```python
from build123d import *

# Parameters (mm, degrees)
SKETCH_1_R          = 0.9
SKETCH_1_W          = 6
SKETCH_1_H          = 8
EXTRUDE_1_DEPTH     = 16.3
SKETCH_2_R          = 0.75
CUT_EXTRUDE_1_DEPTH = 4
CUT_EXTRUDE_START   = -16
SKETCH_2_3_R        = 0.75
CUT_EXTRUDE_2_DEPTH = 4


with BuildPart() as part:
    # 草图1 → 凸台-拉伸1 (new body)
    # profile 1 of 4: a face of its own
    with BuildSketch(Plane.XY):
        Polygon((44, 10), (0, 10), (0, 4), (5, 4), (11, 4), (33, 4), (39, 4), (44, 4), align=None)
        with Locations((8, 7)):
            Circle(SKETCH_1_R, mode=Mode.SUBTRACT)
        with Locations((36, 7)):
            Circle(SKETCH_1_R, mode=Mode.SUBTRACT)
    # profile 2 of 4: a face of its own
    with BuildSketch(Plane.XY):
        Polygon((5, -4), (0, -4), (0, -10), (44, -10), (44, -4), (39, -4), (33, -4), (11, -4), align=None)
        with Locations((8, -7)):
            Circle(SKETCH_1_R, mode=Mode.SUBTRACT)
        with Locations((36, -7)):
            Circle(SKETCH_1_R, mode=Mode.SUBTRACT)
    # profile 3 of 4: a face of its own
    with BuildSketch(Plane.XY):
        with Locations((8, 0)):
            Rectangle(SKETCH_1_W, SKETCH_1_H)
    # profile 4 of 4: a face of its own
    with BuildSketch(Plane.XY):
        with Locations((36, 0)):
            Rectangle(SKETCH_1_W, SKETCH_1_H)
    extrude(amount=EXTRUDE_1_DEPTH)

    # 草图2 → 切除-拉伸1 (cut)
    with BuildSketch(Plane(origin=(0, 10, 0), x_dir=(1, 0, 0), z_dir=(0, 1, 0))):
        with Locations(Location((8.5, -8.15, 0), (0, 0, 180))):
            Circle(SKETCH_2_R)
        with Locations(Location((35.5, -8.15, 0), (0, 0, 180))):
            Circle(SKETCH_2_R)
    extrude(amount=-CUT_EXTRUDE_1_DEPTH, mode=Mode.SUBTRACT)

    # 草图2<3> → 切除-拉伸2 (cut)
    with BuildSketch(Plane(origin=(0, 10, 0), x_dir=(1, 0, 0), z_dir=(0, 1, 0)).offset(CUT_EXTRUDE_START)):
        with Locations(Location((8.5, -8.15, 0), (0, 0, 180))):
            Circle(SKETCH_2_3_R)
        with Locations(Location((35.5, -8.15, 0), (0, 0, 180))):
            Circle(SKETCH_2_3_R)
    extrude(amount=-CUT_EXTRUDE_2_DEPTH, mode=Mode.SUBTRACT)


solid = part.part
```
Geometry check sheet. Reference: the model listing, model coordinates, mm. A direction names the side the tool comes from. Round coordinates to 2 decimals unless told otherwise and drop trailing zeros. Write each loop counter-clockwise with the first axis right and the second up, starting at its lowest first coordinate (ties: lowest second). Pieces come first, ordered by that corner, then holes. Notation, with made-up numbers: (48.25, -25) -> (82.25, -25) arc R20 cw to (82.25, -2) -> close; hole circle Ø1 at (-24.75, 75). An arc over 180 degrees is marked (long way). Put each result on its own line as item: value.
1) Thickness scan on probe 1 along Y at (x, z) = (8, 10.5); probe 2 along Y at (x, z) = (3, 8.5); probe 3 along X at (y, z) = (-3.5, 8). Record the ranges inside material, lowest first. Write a range as from..to.
Recorded:
probe 1: y = -10..-7.9, -6.1..6.1, 7.9..10
probe 2: y = -10..-4, 4..10
probe 3: x = 5..11, 33..39
2) Release check for a two-part mould opening along Z. For faces 4 (the face through (22, 5, 16.3)), 5 (the face through (2, 4, 8)), 6 (the face through (34.785, -8.416, 8.375)) record: pulls with the +Z half, pulls with the -Z half, needs draft (parallel to the pull), parting line crosses it, or undercut.
Recorded:
face 4: pulls with the +Z half
face 5: needs draft
face 6: undercut
3) Cross-section at D-D, the plane y = -7. Enter the section's corners in (x, z), plus the area to 3 significant figures.
Recorded:
outline: (0, 0) -> (7.1, 0) -> (7.1, 16.3) -> (0, 16.3) -> close; (8.9, 0) -> (35.1, 0) -> (35.1, 7.52) arc R0.75 cw to (35.1, 8.78) -> (35.1, 16.3) -> (8.9, 16.3) -> (8.9, 8.78) arc R0.75 cw to (8.9, 7.52) -> close; (36.9, 0) -> (44, 0) -> (44, 16.3) -> (36.9, 16.3) -> close
area: 658 mm2
4) Depth check by flat-ended pin: P1, Ø1.4, axis at x = 35.5, z = 8.15, coming from the +Y side; P2, Ø1.4, axis at x = 8.5, z = 8.15, coming from the -Y side; P3, Ø4, axis at y = 0.5, z = 8, coming from the +X side. Enter the tip coordinate at first touch or a pass-through.
Recorded:
P1: stops at y = 6
P2: stops at y = -6
P3: stops at x = 39
5) Cross-section at B-B, the plane x = 23. Enter the section's corners in (y, z).
Recorded:
outline: (-10, 0) -> (-4, 0) -> (-4, 16.3) -> (-10, 16.3) -> close; (4, 0) -> (10, 0) -> (10, 16.3) -> (4, 16.3) -> close
6) Access from +Z, -Z, +X, -X, +Y, -Y to the whole of each face (thin tool, end or side, straight path). Record for faces 1 (the face through (3, -4, 8)), 2 (the face through (39, 0, 8)), 3 (the face through (22, 4, 8)).
Recorded:
face 1: +Z, -Z, -X
face 2: +Z, -Z, +X
face 3: +Z, -Z
7) Cross-section at A-A, the plane z = 5.5. Enter the section's corners in (x, y).
Recorded:
outline: (0, -10) -> (44, -10) -> (44, -4) -> (39, -4) -> (39, 4) -> (44, 4) -> (44, 10) -> (0, 10) -> (0, 4) -> (5, 4) -> (5, -4) -> (0, -4) -> close; hole circle Ø1.8 at (8, -7); hole circle Ø1.8 at (8, 7); hole (11, -4) -> (33, -4) -> (33, 4) -> (11, 4) -> close; hole circle Ø1.8 at (36, -7); hole circle Ø1.8 at (36, 7)
8) Cross-section at C-C, the plane y = 0.5. Enter the section's corners in (x, z), plus the area to 3 significant figures.
Recorded:
outline: (5, 0) -> (11, 0) -> (11, 16.3) -> (5, 16.3) -> close; (33, 0) -> (39, 0) -> (39, 16.3) -> (33, 16.3) -> close
area: 196 mm2
